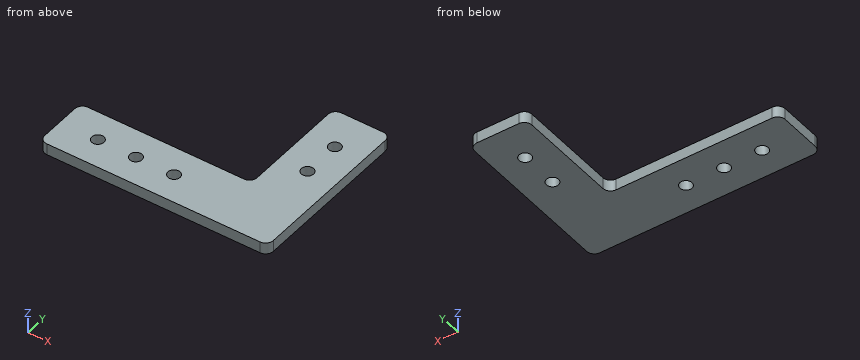
Autodesk Inventor part; units mm, degrees
ref_plane "YZ Plane" through (0, 0, 0) normal (1, 0, 0) x (0, 1, 0)
ref_plane "XZ Plane" through (0, 0, 0) normal (0, 1, 0) x (-1, 0, 0)
ref_plane "XY Plane" through (0, 0, 0) normal (0, 0, 1) x (1, 0, 0)
sketch "スケッチ1" plane through (0, 0, 0) normal (0, 0, 1) x (1, 0, 0)
  line L0 (0, 0) -> (80, 0)
  line L1 (80, 0) -> (80, 45)
  line L2 (80, 45) -> (0, 45)
  line L3 (0, 45) -> (0, 0)
  dimension "d0" = 80
  dimension "d1" = 45
extrude "押し出し1" add sketch "スケッチ1" along normal blind 3
sketch "スケッチ2" plane through (0, 0, 3) normal (0, 0, 1) x (1, 0, 0)
  line L0 (0, 45) -> (0, 0)
  line L1 (0, 0) -> (80, 0)
  line L2 (80, 45) -> (0, 45)
  line L3 (40, 45) -> (40, 0) construction
  point P0 (7.5, 35)
  point P1 (7.5, 25)
  point P2 (30, 7.5)
  point P3 (72.5, 35)
  point P4 (72.5, 25)
  point P5 (50, 7.5)
  point P6 (40, 7.5)
  dimension "d4" = 7.5
  dimension "d5" = 35
  dimension "d6" = 10
  dimension "d7" = 7.5
  dimension "d8" = 7.5
  dimension "d9" = 30
hole "穴1" at (7.5, 35, 3) at (7.5, 25, 3) at (30, 7.5, 3) at (72.5, 35, 3) at (72.5, 25, 3) at (50, 7.5, 3) at (40, 7.5, 3) direction (0, 0, -1) diameter 3.2 end through all
sketch "スケッチ3" plane through (0, 0, 3) normal (0, 0, 1) x (1, 0, 0)
  line L0 (80, 45) -> (0, 45)
  line L1 (15, 45) -> (65, 45)
  line L2 (65, 45) -> (65, 15)
  line L3 (65, 15) -> (15, 15)
  line L4 (15, 15) -> (15, 45)
  line L5 (0, 45) -> (0, 0)
  line L6 (0, 0) -> (80, 0)
  dimension "d17" = 50
  dimension "d18" = 30
  dimension "d19" = 15
  dimension "d20" = 15
extrude "押し出し2" cut sketch "スケッチ3" against normal blind 3
fillet "フィレット1" radius 2 8 edges at (15, 45, 1.5) (65, 15, 1.5) (65, 45, 1.5) (80, 45, 1.5) (0, 45, 1.5) (0, 0, 1.5) (80, 0, 1.5) (15, 15, 1.5)
sketch "スケッチ4" plane through (0, 0, 3) normal (0, 0, 1) x (1, 0, 0)
  line L0 (17, 15) -> (63, 15)
  line L1 (20, 15) -> (20, 0)
  line L2 (2, 0) -> (78, 0)
  circle A0 centre (30, 7.5) radius 1.6
  line L3 (20, 15) -> (14.3834, 55.3393)
  line L4 (14.3834, 55.3393) -> (-4.9194, 44.4595)
  line L5 (-4.9194, 44.4595) -> (-4.9194, 0)
  line L6 (-4.9194, 0) -> (20, 0)
  point P0 (0, 0)
  dimension "d24" = 10
extrude "押し出し3" cut sketch "スケッチ4" against normal blind 10 contours L1 L2 L6 L5 L4 L3
fillet "フィレット2" radius 2 2 edges at (20, 15, 1.5) (20, 0, 1.5)
properties part number "射出_固定6" material "アルミニウム 6061"
Read the model definition and answer for the solid it produces. Units are mm, in the model's axes. Give positions to 0.01 mm unless a question says otherwise; leave off trailing zeros. Order: outer loops, then holes, each group sorted by start corner. A loop starts at its lowest first (then second) coordinate and runs counter-clockwise, first axis right, second up. Notation, with made-up numbers: (-8, -30.5) -> (-4, -30.5) arc R16 ccw to (-4, -6.5) -> close; hole circle Ø8 at (-18, 73). An arc over 180 degrees is marked (long way). Write item = value, one per line.
1. Straight lines are drawn through the part: line 1 along X through (y, z) = (7.5, 2.3); line 2 along Y through (x, z) = (72.5, 0.8); line 3 along Y through (x, z) = (30, 0.9). For each, find the intervals that lie inside material, in ascending order.
Numbers:
line_1 = 20 to 28.4, 31.6 to 38.4, 41.6 to 48.4, 51.6 to 80
line_2 = 0 to 23.4, 26.6 to 33.4, 36.6 to 45
line_3 = 0 to 5.9, 9.1 to 15
2. A cutting plane is placed at A-A, the plane x = 30. Write down the section's boundary in (y, z).
Numbers:
outline = (0, 0) -> (5.9, 0) -> (5.9, 3) -> (0, 3) -> close; (9.1, 0) -> (15, 0) -> (15, 3) -> (9.1, 3) -> close
3. Given pin 1 (1.5 mm diameter, centred on x = 47.5, z = 1, fed in from -Y); pin 2 (0.9 mm diameter, centred on y = 30.5, z = 1.5, fed in from -X), each flat-ended and moving along its own axis, determine where each tip first touches the part or whether it passes through.
Numbers:
pin_1 = 0
pin_2 = 65
4. A cutting plane is placed at C-C, the plane y = 7.5. Write down the section's boundary in (x, z).
Numbers:
outline = (20, 0) -> (28.4, 0) -> (28.4, 3) -> (20, 3) -> close; (31.6, 0) -> (38.4, 0) -> (38.4, 3) -> (31.6, 3) -> close; (41.6, 0) -> (48.4, 0) -> (48.4, 3) -> (41.6, 3) -> close; (51.6, 0) -> (80, 0) -> (80, 3) -> (51.6, 3) -> close
5. A cutting plane is placed at D-D, the plane z = 1.3. Write down the section's boundary in (x, y), and give its area (3 significant figures).
Numbers:
outline = (20, 2) arc R2 ccw to (22, 0) -> (78, 0) arc R2 ccw to (80, 2) -> (80, 43) arc R2 ccw to (78, 45) -> (67, 45) arc R2 ccw to (65, 43) -> (65, 17) arc R2 cw to (63, 15) -> (22, 15) arc R2 ccw to (20, 13) -> close; hole circle Ø3.2 at (30, 7.5); hole circle Ø3.2 at (40, 7.5); hole circle Ø3.2 at (50, 7.5); hole circle Ø3.2 at (72.5, 25); hole circle Ø3.2 at (72.5, 35)
area = 1,310 mm²
6. A cutting plane is placed at B-B, the plane y = 25. Write down the section's boundary in (x, z), and give its area (3 significant figures).
Numbers:
outline = (65, 0) -> (70.9, 0) -> (70.9, 3) -> (65, 3) -> close; (74.1, 0) -> (80, 0) -> (80, 3) -> (74.1, 3) -> close
area = 35.4 mm²
